Drawing for the job (mm, zero at the part's lowest x, y, z). A direction names the side the tool comes from. Round coordinates to 2 decimals unless told otherwise and drop trailing zeros. Write each loop counter-clockwise with the first axis right and the second up, starting at its lowest first coordinate (ties: lowest second). Pieces come first, ordered by that corner, then holes. Notation, with made-up numbers: M -36.5,23 L 10.5,23 A31 ccw 10.5,50 Z; hole C 58,8.5 d6. An arc over 180 degrees is marked long. Use a Markdown table: item, result. Add a question column.
1) Drop flat-ended pins along their axis: P1, Ø8, axis at x = 53.5, y = 2.5, coming from the -Z side; P2, Ø4, axis at x = 58.5, z = 5, coming from the +Y side; P3, Ø1.5, axis at x = 34, z = 4, coming from the +Y side (3 decimals). Give the stop position or say it passes through.
2) Slice it at C-C on z = 5. Write the cut outline in (x, y).
3) Slice it at D-D on y = 1.5. Write the cut outline in (x, z), plus the area to 3 significant figures.
4) Slice it at B-B on y = 7.5. Write the cut outline in (x, z), plus the area to 3 significant figures.
5) Which spindle directions (+Z, -Z, +X, -X, +Y, -Y) get a long thin tool onto all of the face, cutting with end or side? Do the marked faces 1 and 2. Say none if no direction does.
6) Slice it at A-A on x = 58.5. Write the cut outline in (y, z).
7) Wall check: probe 1 along X at (y, z) = (11.5, 5.75); probe 2 along Z at (x, y) = (5, 4); probe 3 along X at (y, z) = (14.5, 6.5). Give the ranges that are in metal, low to high.
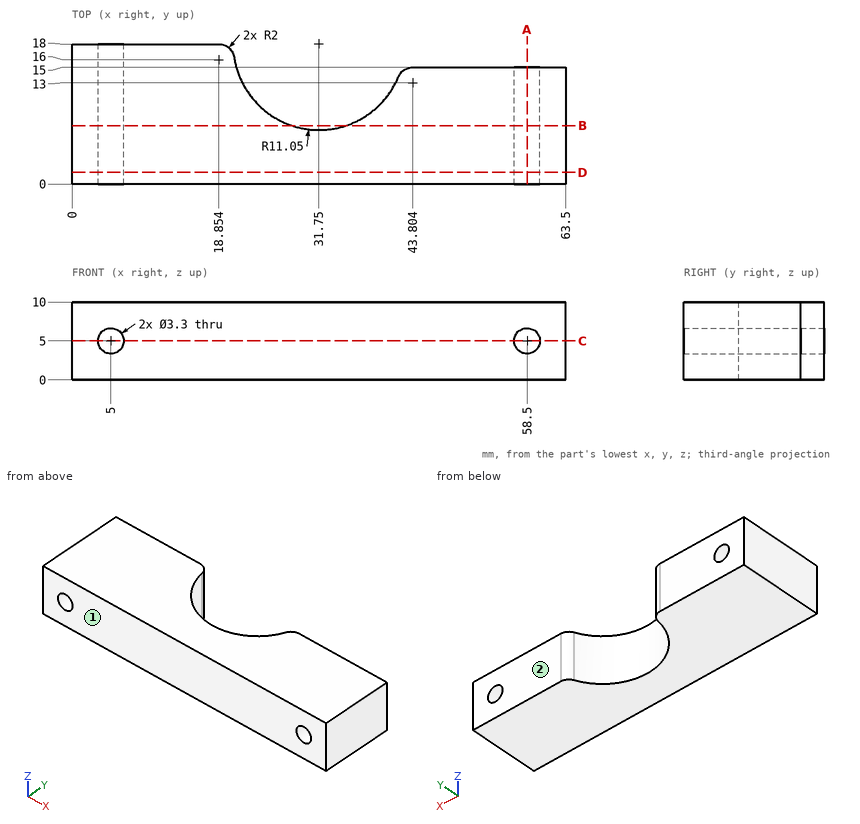
Entries:
| question | item | result |
|---|---|---|
| 1 | P1 | stops at z = 0 |
| 1 | P2 | stops at y = 15 |
| 1 | P3 | stops at y = 7.365 |
| 2 | outline | M 0,0 L 3.35,0 L 3.35,18 L 0,18 Z; M 6.65,0 L 56.85,0 L 56.85,15 L 43.8,15 A2 ccw 41.96,13.77 A11.05 cw 20.83,16.31 A2 ccw 18.85,18 L 6.65,18 Z; M 60.15,0 L 63.5,0 L 63.5,15 L 60.15,15 Z |
| 3 | outline | M 0,0 L 63.5,0 L 63.5,10 L 0,10 Z; hole C 5,5 d3.3; hole C 58.5,5 d3.3 |
| 3 | area | 618 mm^2 |
| 4 | outline | M 0,0 L 28.31,0 L 28.31,10 L 0,10 Z; M 35.19,0 L 63.5,0 L 63.5,10 L 35.19,10 Z; hole C 5,5 d3.3; hole C 58.5,5 d3.3 |
| 4 | area | 549 mm^2 |
| 5 | face 1 | +Z, -Z, +X, -X, -Y |
| 5 | face 2 | +Z, -Z, +X, +Y |
| 6 | outline | M 0,0 L 15,0 L 15,3.35 L 0,3.35 Z; M 0,6.65 L 15,6.65 L 15,10 L 0,10 Z |
| 7 | probe 1 | x = 0 to 3.53, 6.47 to 22.81, 40.69 to 57.03, 59.97 to 63.5 |
| 7 | probe 2 | z = 0 to 3.35, 6.65 to 10 |
| 7 | probe 3 | x = 0 to 4.31, 5.69 to 21.27, 42.48 to 57.81, 59.19 to 63.5 |
